Input: part model. Units: mm. Frame: model coordinates. A direction names the side the tool comes from. Give positions to 0.01 mm unless a question says otherwise; leave off trailing zeros. Loops run counter-clockwise (first coordinate to the right, second up) from the corner with the lowest first, then second, coordinate; pieces in that order, holes last. Notation, with made-up numbers: (88.5, 50) -> (143.5, 50) arc R32 cw to (143.5, 76) -> close; hole circle Ø5 at (-2.75, 56.5). An arc over 180 degrees is marked (long way). Answer in a Markdown table with one row per item. Add a question column.
```python
from build123d import *

# Parameters (mm, degrees)
CROQUIS1_W                      = 90
CROQUIS1_H                      = 90
CROQUIS1_R                      = 2.5
CROQUIS1_R_2                    = 1.625
CROQUIS1_W_2                    = 23.18
CROQUIS1_H_2                    = 23.18
SALIENTE_EXTRUIR1_DEPTH         = 3
CROQUIS2_R                      = 3.35997123
CORTAR_EXTRUIR1_DEPTH           = 1.8
CORTAR_EXTRUIR1_DRAFT           = -44
CORTAR_EXTRUIR1_PROFILE_2_DEPTH = 1.8
CORTAR_EXTRUIR1_PROFILE_2_DRAFT = -44
CORTAR_EXTRUIR1_PROFILE_3_DEPTH = 1.8
CORTAR_EXTRUIR1_PROFILE_3_DRAFT = -44
CORTAR_EXTRUIR1_PROFILE_4_DEPTH = 1.8
CORTAR_EXTRUIR1_PROFILE_4_DRAFT = -44


with BuildPart() as part:
    # Croquis1 → Saliente-Extruir1 (new body)
    with BuildSketch(Plane.XY):
        with Locations((6.790535393, -1.76108936)):
            Rectangle(CROQUIS1_W, CROQUIS1_H)
        with Locations((-30.272299079, 19.584790813)):
            Circle(CROQUIS1_R, mode=Mode.SUBTRACT)
        with Locations((-30.262724761, 12.486512925)):
            Circle(CROQUIS1_R, mode=Mode.SUBTRACT)
        with Locations((-29.209464607, 34.23891064)):
            Circle(CROQUIS1_R_2, mode=Mode.SUBTRACT)
        with Locations((19.459089133, 34.23891064)):
            Circle(CROQUIS1_R_2, mode=Mode.SUBTRACT)
        with Locations((-29.209464607, -37.76108936)):
            Circle(CROQUIS1_R_2, mode=Mode.SUBTRACT)
        with Locations((19.459089133, -37.76108936)):
            Circle(CROQUIS1_R_2, mode=Mode.SUBTRACT)
        with Locations((6.790535393, -1.76108936)):
            Rectangle(CROQUIS1_W_2, CROQUIS1_H_2, mode=Mode.SUBTRACT)
        with BuildLine():
            Line((-11.293405686, 27.67391064), (-11.293405686, 16.17391064))
            ThreePointArc((-11.293405686, 16.17391064), (-12.043405686, 15.42391064), (-12.793405686, 16.17391064))
            Line((-12.793405686, 16.17391064), (-12.793405686, 27.67391064))
            ThreePointArc((-12.793405686, 27.67391064), (-12.043405686, 28.42391064), (-11.293405686, 27.67391064))
        make_face(mode=Mode.SUBTRACT)
        with BuildLine():
            Line((-14.308998248, 26.794100575), (-14.308998248, 17.053720706))
            ThreePointArc((-14.308998248, 17.053720706), (-15.058998248, 16.303720706), (-15.808998248, 17.053720706))
            Line((-15.808998248, 17.053720706), (-15.808998248, 26.794100575))
            ThreePointArc((-15.808998248, 26.794100575), (-15.058998248, 27.544100575), (-14.308998248, 26.794100575))
        make_face(mode=Mode.SUBTRACT)
        with BuildLine():
            Line((-8.210041057, 26.794100575), (-8.210041057, 17.053720706))
            ThreePointArc((-8.210041057, 17.053720706), (-8.960041057, 16.303720706), (-9.710041057, 17.053720706))
            Line((-9.710041057, 17.053720706), (-9.710041057, 26.794100575))
            ThreePointArc((-9.710041057, 26.794100575), (-8.960041057, 27.544100575), (-8.210041057, 26.794100575))
        make_face(mode=Mode.SUBTRACT)
        with BuildLine():
            Line((-16.889510612, 23.96392892), (-16.889510612, 19.883892361))
            ThreePointArc((-16.889510612, 19.883892361), (-17.639510612, 19.133892361), (-18.389510612, 19.883892361))
            Line((-18.389510612, 19.883892361), (-18.389510612, 23.96392892))
            ThreePointArc((-18.389510612, 23.96392892), (-17.639510612, 24.71392892), (-16.889510612, 23.96392892))
        make_face(mode=Mode.SUBTRACT)
        with BuildLine():
            Line((-5.604418602, 23.96392892), (-5.604418602, 19.883892361))
            ThreePointArc((-5.604418602, 19.883892361), (-6.354418602, 19.133892361), (-7.104418602, 19.883892361))
            Line((-7.104418602, 19.883892361), (-7.104418602, 23.96392892))
            ThreePointArc((-7.104418602, 23.96392892), (-6.354418602, 24.71392892), (-5.604418602, 23.96392892))
        make_face(mode=Mode.SUBTRACT)
    extrude(amount=SALIENTE_EXTRUIR1_DEPTH)


with BuildPart() as cortar_extruir1_tool:
    # Croquis2 → Cortar-Extruir1 (with draft: the straight prism first)
    with BuildSketch(Plane.XY.offset(3)):
        with Locations((-29.209464607, 34.23891064)):
            Circle(CROQUIS2_R)
    extrude(amount=-CORTAR_EXTRUIR1_DEPTH)
    # Cortar-Extruir1: the draft: its side faces are tilted about the plane it starts from
    cortar_extruir1_sides = [cortar_extruir1_tool.faces().sort_by_distance(p)[0] for p in [
        (-32.569435837, 34.23891064, 2.1),
    ]]
    draft(cortar_extruir1_sides, Plane.XY.offset(3), CORTAR_EXTRUIR1_DRAFT)


with BuildPart() as part_1:
    add(part.part)

    # Cortar-Extruir1: cut by cortar_extruir1_tool
    add(cortar_extruir1_tool.part, mode=Mode.SUBTRACT)


with BuildPart() as cortar_extruir1_profile_2_tool:
    # Croquis2 → Cortar-Extruir1 profile 2 (with draft: the straight prism first)
    with BuildSketch(Plane.XY.offset(3)):
        with Locations((19.459089133, 34.23891064)):
            Circle(CROQUIS2_R)
    extrude(amount=-CORTAR_EXTRUIR1_PROFILE_2_DEPTH)
    # Cortar-Extruir1 profile 2: the draft: its side faces are tilted about the plane it starts from
    cortar_extruir1_profile_2_sides = [cortar_extruir1_profile_2_tool.faces().sort_by_distance(p)[0] for p in [
        (16.099117903, 34.23891064, 2.1),
    ]]
    draft(cortar_extruir1_profile_2_sides, Plane.XY.offset(3), CORTAR_EXTRUIR1_PROFILE_2_DRAFT)


with BuildPart() as part_2:
    add(part_1.part)

    # Cortar-Extruir1 profile 2: cut by cortar_extruir1_profile_2_tool
    add(cortar_extruir1_profile_2_tool.part, mode=Mode.SUBTRACT)


with BuildPart() as cortar_extruir1_profile_3_tool:
    # Croquis2 → Cortar-Extruir1 profile 3 (with draft: the straight prism first)
    with BuildSketch(Plane.XY.offset(3)):
        with Locations((19.459089133, -37.76108936)):
            Circle(CROQUIS2_R)
    extrude(amount=-CORTAR_EXTRUIR1_PROFILE_3_DEPTH)
    # Cortar-Extruir1 profile 3: the draft: its side faces are tilted about the plane it starts from
    cortar_extruir1_profile_3_sides = [cortar_extruir1_profile_3_tool.faces().sort_by_distance(p)[0] for p in [
        (16.099117903, -37.76108936, 2.1),
    ]]
    draft(cortar_extruir1_profile_3_sides, Plane.XY.offset(3), CORTAR_EXTRUIR1_PROFILE_3_DRAFT)


with BuildPart() as part_3:
    add(part_2.part)

    # Cortar-Extruir1 profile 3: cut by cortar_extruir1_profile_3_tool
    add(cortar_extruir1_profile_3_tool.part, mode=Mode.SUBTRACT)


with BuildPart() as cortar_extruir1_profile_4_tool:
    # Croquis2 → Cortar-Extruir1 profile 4 (with draft: the straight prism first)
    with BuildSketch(Plane.XY.offset(3)):
        with Locations((-29.209464607, -37.76108936)):
            Circle(CROQUIS2_R)
    extrude(amount=-CORTAR_EXTRUIR1_PROFILE_4_DEPTH)
    # Cortar-Extruir1 profile 4: the draft: its side faces are tilted about the plane it starts from
    cortar_extruir1_profile_4_sides = [cortar_extruir1_profile_4_tool.faces().sort_by_distance(p)[0] for p in [
        (-32.569435837, -37.76108936, 2.1),
    ]]
    draft(cortar_extruir1_profile_4_sides, Plane.XY.offset(3), CORTAR_EXTRUIR1_PROFILE_4_DRAFT)


with BuildPart() as part_4:
    add(part_3.part)

    # Cortar-Extruir1 profile 4: cut by cortar_extruir1_profile_4_tool
    add(cortar_extruir1_profile_4_tool.part, mode=Mode.SUBTRACT)


solid = part_4.part
```
1) Reachability of faces 1 (the face through (-16.89, 22, 1)), 2 (the face through (-27.556, 34.76, 1.316)) from +Z, -Z, +X, -X, +Y, -Y: full face, straight path, thin tool, end or side. Return the list, or none.
2) Pin query (flat end, axial travel): pin 1 (1.5 mm diameter, centred on x = 37.5, y = -2, fed in from -Z); pin 2 (2.5 mm diameter, centred on x = 19.46, y = -37.76, fed in from +Z). Return the tip coordinate at first contact, or that it passes through.
3) Section B-B on y = 1. Output: boundary loops of the cut face in (x, z), and give its area (3 significant figures).
4) Section A-A on x = 1.5. Output: boundary loops of the cut face in (y, z), and give its area (3 significant figures).
5) Section C-C on z = 1.7. State how many separate pieces and enclosed holes the cut face has, and give its area (3 significant figures).
6) Pull-direction query (Y, two-part tool) for faces 3 (the face through (6, -46.761, 1)), 4 (the face through (26, -1, 0)), 5 (the face through (-28.278, -36.299, 1.316)), 6 (the face through (18.261, -36.663, 0.593)); classes: +Y half, -Y half, draft (parallel to the pull), parting line (faces both ways), or undercut.
7) Material intervals for line 1 along X through (y, z) = (34.5, 1.1); line 2 along X through (y, z) = (5.5, 0.15); line 3 along X through (y, z) = (-36, 2.5), sorted ascending.
Working result:
| question | item | result |
|---|---|---|
| 1 | face 1 | +Z, -Z |
| 1 | face 2 | +Z |
| 2 | pin 1 | stops at z = 0 |
| 2 | pin 2 | passes through |
| 3 | outline | (-38.21, 0) -> (-4.8, 0) -> (-4.8, 3) -> (-38.21, 3) -> close; (18.38, 0) -> (51.79, 0) -> (51.79, 3) -> (18.38, 3) -> close |
| 3 | area | 200 mm2 |
| 4 | outline | (-46.76, 0) -> (-13.35, 0) -> (-13.35, 3) -> (-46.76, 3) -> close; (9.83, 0) -> (43.24, 0) -> (43.24, 3) -> (9.83, 3) -> close |
| 4 | area | 200 mm2 |
| 5 | separate pieces | 1 |
| 5 | enclosed holes | 12 |
| 5 | area | 7,400 mm2 |
| 6 | face 3 | -Y half |
| 6 | face 4 | draft |
| 6 | face 5 | undercut |
| 6 | face 6 | undercut |
| 7 | line 1 | x = -38.21 to -30.81, -27.61 to 17.86, 21.06 to 51.79 |
| 7 | line 2 | x = -38.21 to -4.8, 18.38 to 51.79 |
| 7 | line 3 | x = -38.21 to -31.48, -26.93 to 17.18, 21.73 to 51.79 |
